Model file for the job. Use its own axes, mm. A direction names the side the tool comes from. Give positions to 0.01 mm unless a question says otherwise; leave off trailing zeros. Write each loop counter-clockwise with the first axis right and the second up, starting at its lowest first coordinate (ties: lowest second). Pieces come first, ordered by that corner, then holes.
```python
from build123d import *

# Parameters (mm, degrees)
SKETCH1_R           = 25
BOSS_EXTRUDE1_DEPTH = 10
SKETCH2_R           = 15
BOSS_EXTRUDE2_DEPTH = 10
SKETCH3_W           = 10
SKETCH3_H           = 10
BOSS_EXTRUDE3_DEPTH = 2


with BuildPart() as part:
    # Sketch1 → Boss-Extrude1 (new body)
    with BuildSketch(Plane(origin=(0, 0, 0), x_dir=(1, 0, 0), z_dir=(0, 1, 0))):
        with Locations(Location((0, 0, 0), (0, 0, 270))):
            Circle(SKETCH1_R)
    extrude(amount=BOSS_EXTRUDE1_DEPTH)

    # Sketch2 → Boss-Extrude2 (add)
    with BuildSketch(Plane(origin=(0, 10, 0), x_dir=(1, 0, 0), z_dir=(0, 1, 0))):
        with Locations(Location((0, 0, 0), (0, 0, 270))):
            Circle(SKETCH2_R)
    extrude(amount=BOSS_EXTRUDE2_DEPTH)

    # Sketch3 → Boss-Extrude3 (add)
    with BuildSketch(Plane.XZ):
        Rectangle(SKETCH3_W, SKETCH3_H)
    extrude(amount=BOSS_EXTRUDE3_DEPTH)


solid = part.part
```
1. Slice it at A-A, the plane z = 0. Write the cut outline in (x, y).
Calculated:
outline: (-25, 0) - (-5, 0) - (-5, -2) - (5, -2) - (5, 0) - (25, 0) - (25, 10) - (15, 10) - (15, 20) - (-15, 20) - (-15, 10) - (-25, 10) - close
2. Slice it at D-D, the plane x = -10. Write the cut outline in (y, z), and give its area (3 significant figures).
Calculated:
outline: (0, -22.91) - (10, -22.91) - (10, -11.18) - (20, -11.18) - (20, 11.18) - (10, 11.18) - (10, 22.91) - (0, 22.91) - close
area: 682 mm2
3. Slice it at B-B, the plane x = 0. Write the cut outline in (y, z), and give its area (3 significant figures).
Calculated:
outline: (-2, -5) - (0, -5) - (0, -25) - (10, -25) - (10, -15) - (20, -15) - (20, 15) - (10, 15) - (10, 25) - (0, 25) - (0, 5) - (-2, 5) - close
area: 820 mm2
4. Pin check, flat tips, straight feed: P1, Ø1, axis at x = -3, y = 9.5, coming from the -Z side; P2, Ø1.5, axis at y = 6, z = 19, coming from the +X side; P3, Ø4, axis at y = 10.5, z = 15, coming from the +X side. Stop position of each tip, or through.
Calculated:
P1: stops at z = -24.87
P2: stops at x = 17.09
P3: stops at x = 21.32
5. Which spindle directions (+Z, -Z, +X, -X, +Y, -Y) get a long thin tool onto all of the face, cutting with end or side? Do faces 1 (the flat face through (5, -1, 0)), 2 (the flat face through (0, -1, 5)), 3 (the flat face through (-11, 10, 11)). Say none if no direction does.
Calculated:
face 1: +Z, -Z, +X, -Y
face 2: +Z, +X, -X, -Y
face 3: +Y
6. Probe probe 1 along Y at (x, z) = (-3, -18.5); probe 2 along X at (y, z) = (16.25, 0); probe 3 along Y at (x, z) = (-0.5, -7). List the from-to ranges inside material, lowest first.
Calculated:
probe 1: y = 0 to 10
probe 2: x = -15 to 15
probe 3: y = 0 to 20
7. Slice it at C-C, the plane y = 13. Write the cut outline in (x, z).
Calculated:
outline: circle Ø30 at (0, 0)
